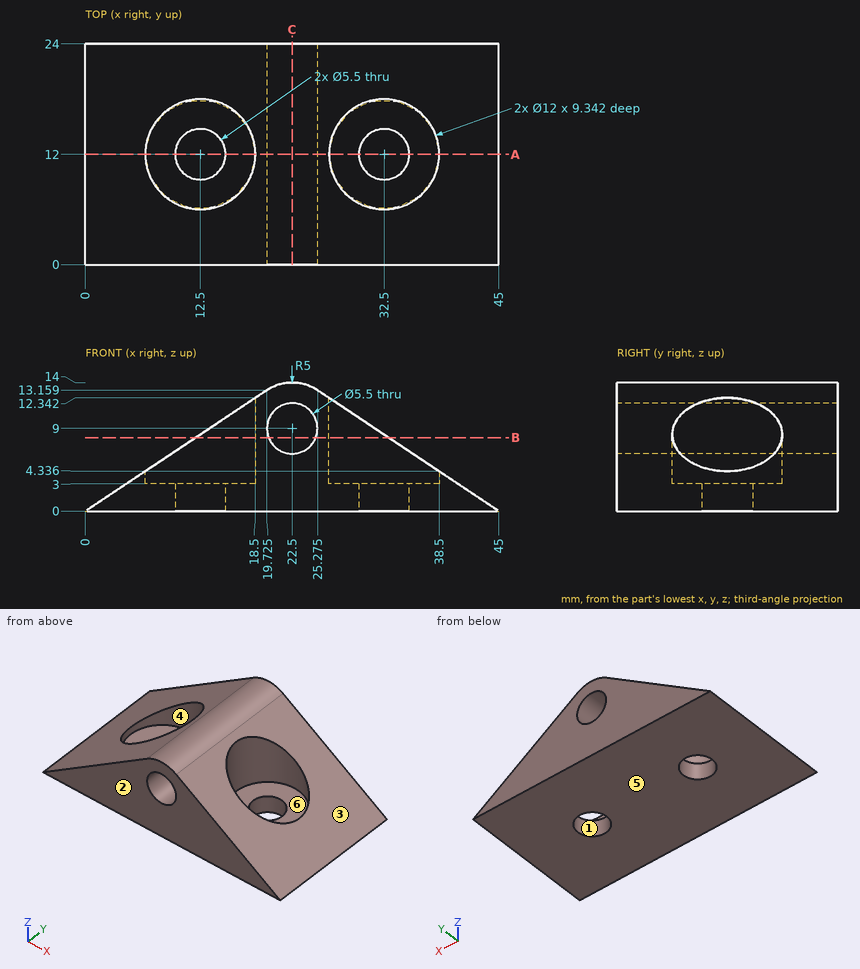
For this review, use the dimensioned drawing (mm, ordinates from the lowest corner) and the shaded views. A direction names the side the tool comes from. Give positions to 0.01 mm unless a question says otherwise; leave off trailing zeros. Order: outer loops, then holes, each group sorted by start corner. A loop starts at its lowest first (then second) coordinate and runs counter-clockwise, first axis right, second up. Notation, with made-up numbers: (43.5, 13.5) - (83.5, 13.5) arc R10 cw to (83.5, 20.5) - close; hole circle Ø10 at (-18.75, 68.5). An arc over 180 degrees is marked (long way). Use a Markdown table: item, result. Add a question column.
(1) Add section A-A on y = 12. Give the number of separate pieces and of enclosed holes in the cut face, then the cut area to 3 significant figures.
(2) Add section C-C on x = 22.5. Give the boundary of the cut face in (y, z), then the cut area to 3 significant figures.
(3) Wall thickness on probe 1 along Y at (x, z) = (32.5, 5.75); probe 2 along Y at (x, z) = (12.5, 1.4); probe 3 along Z at (x, y) = (22.5, 10.25): over which ranges is each line inside the solid? List them lowest first. Write a range as [from, to].
(4) Machinability: for the marked faces 5 and 6, which of the approach directions +Z, -Z, +X, -X, +Y, -Y give a long, thin tool a straight path to every point of the face, cutting with its end or side? Answer none if there is none.
(5) Mouldability with a two-part tool opening along Y and no side actions: class the marked faces 1, 2, 3 and 4 as +Y half, -Y half, draft (parallel to the pull), parting line (faces both ways), or undercut.
(6) Add section B-B on z = 8. Give the boundary of the cut face in (x, y), then the cut area to 3 significant figures.
(7) Clearance check with flat-ended pins moving along their axes: P1, Ø13, axis at x = 34, y = 9.5, coming from the +Z side; P2, Ø9, axis at x = 12.5, y = 12, coming from the +Z side; P3, Ø1, axis at y = 8, z = 4.5, coming from the -X side (1 decimal). State where each tip first meets the part, or that it passes through.
Report:
| question | item | result |
|---|---|---|
| 1 | separate pieces | 3 |
| 1 | enclosed holes | 1 |
| 1 | area | 151 mm² |
| 2 | outline | (0, 0) - (24, 0) - (24, 6.25) - (0, 6.25) - close; (0, 11.75) - (24, 11.75) - (24, 14) - (0, 14) - close |
| 2 | area | 204 mm² |
| 3 | probe 1 | y = [0, 6], [18, 24] |
| 3 | probe 2 | y = [0, 9.25], [14.75, 24] |
| 3 | probe 3 | z = [0, 6.25], [11.75, 14] |
| 4 | face 5 | -Z, +X, -X, +Y, -Y |
| 4 | face 6 | +Z |
| 5 | face 1 | undercut |
| 5 | face 2 | -Y half |
| 5 | face 3 | draft |
| 5 | face 4 | undercut |
| 6 | outline | (11.99, 0) - (19.94, 0) - (19.94, 24) - (11.99, 24) - (11.99, 17.98) arc R6 cw (long way) to (11.99, 6.02) - close; (25.06, 0) - (33.01, 0) - (33.01, 6.02) arc R6 cw (long way) to (33.01, 17.98) - (33.01, 24) - (25.06, 24) - close |
| 6 | area | 256 mm² |
| 7 | P1 | stops at z = 11.63 |
| 7 | P2 | stops at z = 3 |
| 7 | P3 | stops at x = 6 |
